Can you work these out from the model? Positions are in its coordinate system, mm. A direction names the side the tool comes from. Give positions to 0.01 mm unless a question says otherwise; leave off trailing zeros. Order: outer loops, then holes, each group sorted by start corner. A loop starts at its lowest first (then second) coordinate and runs counter-clockwise, first axis right, second up. Notation, with made-up numbers: (31.5, 21.5) -> (73.5, 21.5) arc R17 ccw to (73.5, 46.5) -> close; hole circle Ø4 at (8, 54). An arc over 180 degrees is marked (long way). Answer as CSV lines item,"result".
```python
from build123d import *

# Parameters (mm, degrees)
F0_R     = 19.5
F0_R_2   = 17.5
F1_DEPTH = 30
F2_R     = 24
F2_R_2   = 19.5
F2_R_3   = 17.5
F3_DEPTH = 10
F4_R     = 20
F4_R_2   = 17.5
F5_DEPTH = 80
F6_R     = 24
F6_R_2   = 17.5
F7_DEPTH = 50


# Not quite as in the source:
# - a fillet or chamfer that OpenCascade refuses, or shapes differently, is made with other operations: its cross-section is extruded or revolved along the edge and cut away or added


with BuildPart() as f1:
    # F0 (on Top) → F1 (new body)
    with BuildSketch(Plane.XY):
        Circle(F0_R)
        Circle(F0_R_2, mode=Mode.SUBTRACT)
    extrude(amount=F1_DEPTH)

    # F2 (on face) → F3 (join)
    with BuildSketch(Plane.XY.offset(30)):
        Circle(F2_R)
        Circle(F2_R_2, mode=Mode.SUBTRACT)
        Circle(F2_R_2)
        Circle(F2_R_3, mode=Mode.SUBTRACT)
    extrude(amount=F3_DEPTH)

    # F4 (on face) → F5 (join)
    with BuildSketch(Plane.XY.offset(40)):
        Circle(F4_R)
        Circle(F4_R_2, mode=Mode.SUBTRACT)
    extrude(amount=F5_DEPTH)

    # F6 (on face) → F7 (join)
    with BuildSketch(Plane.XY.offset(120)):
        Circle(F6_R)
        Circle(F6_R_2, mode=Mode.SUBTRACT)
    extrude(amount=F7_DEPTH)

    # F8: fillet of radius 5 on 5 edges, made by hand

    # F8_s1 → F8_t2 (revolve, cut)
    with BuildSketch(Plane.XZ):
        with BuildLine():
            ThreePointArc((24, 165), (22.5355339059, 168.5355339059), (19, 170))
            Line((19, 170), (24, 170))
            Line((24, 170), (24, 165))
        make_face()
    revolve(axis=Axis((0, 0, 170), (0, 0, 1)), mode=Mode.SUBTRACT)

    # F8_s3 → F8_t4 (revolve, cut)
    with BuildSketch(Plane.XZ):
        with BuildLine():
            ThreePointArc((20, 120), (22.8729833462, 121.7367018254), (24, 124.8989794856))
            Line((24, 124.8989794856), (24, 120))
            Line((24, 120), (20, 120))
        make_face()
    revolve(axis=Axis((0, 0, 120), (0, 0, 1)), mode=Mode.SUBTRACT)

    # F8_s5 → F8_t6 (revolve, cut)
    with BuildSketch(Plane.XZ):
        with BuildLine():
            ThreePointArc((24, 35.1010205144), (22.8729833462, 38.2632981746), (20, 40))
            Line((20, 40), (24, 40))
            Line((24, 40), (24, 35.1010205144))
        make_face()
    revolve(axis=Axis((0, 0, 40), (0, 0, 1)), mode=Mode.SUBTRACT)

    # F8_s7 → F8_t8 (revolve, cut)
    with BuildSketch(Plane.XZ):
        with BuildLine():
            ThreePointArc((19.5, 30), (22.7080992435, 31.6208352193), (24, 34.9749371855))
            Line((24, 34.9749371855), (24, 30))
            Line((24, 30), (19.5, 30))
        make_face()
    revolve(axis=Axis((0, 0, 30), (0, 0, 1)), mode=Mode.SUBTRACT)

    # F8_s9 → F8_t10 (revolve, cut)
    with BuildSketch(Plane.XZ):
        with BuildLine():
            ThreePointArc((19.5, 4), (18.972135955, 1.7639320225), (17.5, 0))
            Line((17.5, 0), (19.5, 0))
            Line((19.5, 0), (19.5, 4))
        make_face()
    revolve(axis=Axis((0, 0, 0), (0, 0, 1)), mode=Mode.SUBTRACT)


solid = f1.part
```
Item 1: Please list where these lines run through material, in increasing order: line 1 along Y through (x, z) = (0, 66.5); line 2 along X through (y, z) = (9, 20.5); line 3 along X through (y, z) = (-10, 13).
Numbers:
line 1,"y = -20 to -17.5, 17.5 to 20"
line 2,"x = -17.3 to -15.01, 15.01 to 17.3"
line 3,"x = -16.74 to -14.36, 14.36 to 16.74"
Item 2: For faces 1 (the cylindrical face through (-4.336, -19.524, 79.44)), 2 (the cylindrical face through (-23.977, 1.055, 144.669)), which set-ups out of +Z, -Z, +X, -X, +Y, -Y let a thin tool reach every point of the face, with its end or its side?
Numbers:
face 1,"none"
face 2,"+Z, -Z"
Item 3: Imagine slicing it at A-A, the plane y = 0. Please give me the cut outline in (x, z).
Numbers:
outline,"(-24, 34.97) arc R5 ccw to (-19.5, 30) -> (-19.5, 4) arc R5 ccw to (-17.5, 0) -> (-17.5, 170) -> (-19, 170) arc R5 ccw to (-24, 165) -> (-24, 124.9) arc R5 ccw to (-20, 120) -> (-20, 40) arc R5 ccw to (-24, 35.1) -> close; (17.5, 0) arc R5 ccw to (19.5, 4) -> (19.5, 30) arc R5 ccw to (24, 34.97) -> (24, 35.1) arc R5 ccw to (20, 40) -> (20, 120) arc R5 ccw to (24, 124.9) -> (24, 165) arc R5 ccw to (19, 170) -> (17.5, 170) -> close"
Item 4: We'd pull the mould along Y, two halves only. Please class faces 3 (the cylindrical face through (-13.887, -10.648, 83.81)), 4 (the flat face through (6, -17, 170)), 5 (the cylindrical face through (-2.539, 19.334, 16.818)): released by +Y, released by -Y, zero draft, split by the parting line, or undercut.
Numbers:
face 3,"undercut"
face 4,"zero draft"
face 5,"split by the parting line"
Item 5: Imagine slicing it at C-C, the plane z = 78. Please give me the cut outline in (x, y), then the cut area to 3 significant figures.
Numbers:
outline,"circle Ø40 at (0, 0); hole circle Ø35 at (0, 0)"
area,"295 mm²"
Item 6: For pin 1 (2 mm diameter, centred on y = 12, z = 68.5, fed in from -X); pin 2 (4 mm diameter, centred on x = -18, z = 31.5, fed in from -Y); pin 3 (4 mm diameter, centred on y = -16, z = 52.5, fed in from -X), each with a flat end and sliding along its axis, tell me the tip position at first contact or that it passes through.
Numbers:
pin 1,"stops at x = -16.7"
pin 2,"stops at y = -16.76"
pin 3,"stops at x = -14.28"
Item 7: Imagine slicing it at D-D, the plane z = 149.5. Please give me the cut outline in (x, y), then the cut area to 3 significant figures.
Numbers:
outline,"circle Ø48 at (0, 0); hole circle Ø35 at (0, 0)"
area,"847 mm²"
